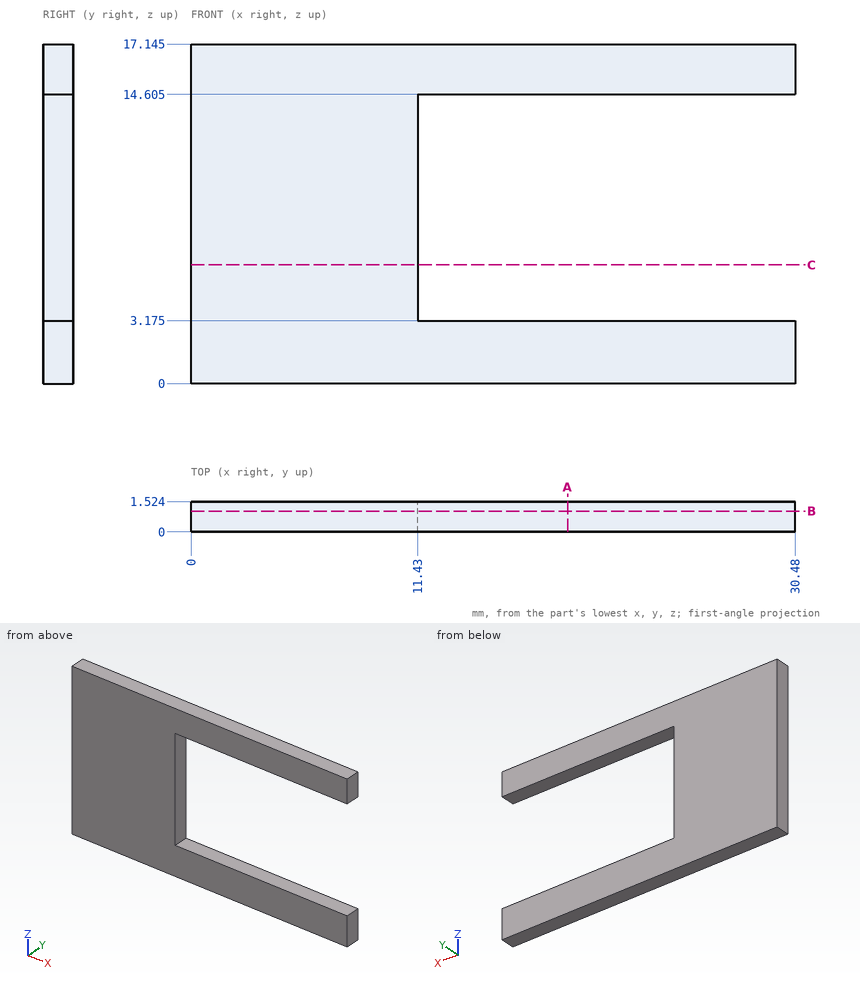
Part print with two shaded views. Sizes in mm from the minimum x, y, z corner. Round coordinates to 2 decimals unless told otherwise and drop trailing zeros. Write each loop counter-clockwise with the first axis right and the second up, starting at its lowest first coordinate (ties: lowest second). Pieces come first, ordered by that corner, then holes. Notation, with made-up numbers: (21.25, 63) - (33.25, 63) arc R24 ccw to (33.25, 99) - close; hole circle Ø6 at (42.5, 85.25). An arc over 180 degrees is marked (long way). Use CSV: the item, a comma, the result in double quotes.
Item 1: Wall check: L1, parallel to Z at x = 18, y = 1.05 (3 decimals); L2, parallel to X at y = 1.05, z = 7.75. Give the ranges that are in metal, low to high.
Results list:
L1,"z = 0 to 3.175, 14.605 to 17.145"
L2,"x = 0 to 11.43"
Item 2: Slice it at A-A, the plane x = 19. Write the cut outline in (y, z) (3 decimals), then the cut area to 3 significant figures.
Results list:
outline,"(0, 0) - (1.524, 0) - (1.524, 3.175) - (0, 3.175) - close; (0, 14.605) - (1.524, 14.605) - (1.524, 17.145) - (0, 17.145) - close"
area,"8.71 mm²"
Item 3: Slice it at B-B, the plane y = 1.05. Write the cut outline in (x, z) (3 decimals).
Results list:
outline,"(0, 0) - (30.48, 0) - (30.48, 3.175) - (11.43, 3.175) - (11.43, 14.605) - (30.48, 14.605) - (30.48, 17.145) - (0, 17.145) - close"
Item 4: Slice it at C-C, the plane z = 6. Write the cut outline in (x, y), then the cut area to 3 significant figures.
Results list:
outline,"(0, 0) - (11.43, 0) - (11.43, 1.52) - (0, 1.52) - close"
area,"17.4 mm²"
